from build123d import *

# Parameters (mm, degrees)
SKETCH_1_W          = 20
SKETCH_1_H          = 15
SKETCH_1_W_2        = 18
SKETCH_1_H_2        = 13
EXTRUDE_1_DEPTH     = 200
SKETCH_3_R          = 1.6
CUT_EXTRUDE_1_DEPTH = 202.137390855
SKETCH_4_R          = 1.6
CUT_EXTRUDE_2_DEPTH = 202.137390855


with BuildPart() as part:
    # 草图1 → 拉伸-薄壁1 (new body)
    with BuildSketch(Plane(origin=(0, 0, 0), x_dir=(1, 0, 0), z_dir=(0, 1, 0))):
        Rectangle(SKETCH_1_W, SKETCH_1_H)
        Rectangle(SKETCH_1_W_2, SKETCH_1_H_2, mode=Mode.SUBTRACT)
    extrude(amount=EXTRUDE_1_DEPTH)

    # 草图3 → 切除-拉伸1 (cut, through all)
    with BuildSketch(Plane(origin=(10, 0, 0), x_dir=(0, 0, -1), z_dir=(1, 0, 0))):
        with Locations((-3.75, 142.5)):
            Circle(SKETCH_3_R)
        with Locations((-3.75, 127.5)):
            Circle(SKETCH_3_R)
        with Locations((3.75, 127.5)):
            Circle(SKETCH_3_R)
        with Locations((3.75, 142.5)):
            Circle(SKETCH_3_R)
        with Locations((-3.75, 72.5)):
            Circle(SKETCH_3_R)
        with Locations((3.75, 72.5)):
            Circle(SKETCH_3_R)
        with Locations((3.75, 57.5)):
            Circle(SKETCH_3_R)
        with Locations((-3.75, 57.5)):
            Circle(SKETCH_3_R)
    extrude(amount=-CUT_EXTRUDE_1_DEPTH, mode=Mode.SUBTRACT)

    # 草图4 → 切除-拉伸2 (cut, through all)
    with BuildSketch(Plane(origin=(10, 0, 0), x_dir=(0, 0, -1), z_dir=(1, 0, 0))):
        with Locations((-3.75, 5)):
            Circle(SKETCH_4_R)
        with Locations((-3.75, 15)):
            Circle(SKETCH_4_R)
        with Locations((3.75, 5)):
            Circle(SKETCH_4_R)
        with Locations((3.75, 15)):
            Circle(SKETCH_4_R)
        with Locations((3.75, 185)):
            Circle(SKETCH_4_R)
        with Locations((3.75, 195)):
            Circle(SKETCH_4_R)
        with Locations((-3.75, 185)):
            Circle(SKETCH_4_R)
        with Locations((-3.75, 195)):
            Circle(SKETCH_4_R)
    extrude(amount=-CUT_EXTRUDE_2_DEPTH, mode=Mode.SUBTRACT)


solid = part.part
The model under review builds one solid part; all positions refer to its coordinate system, in mm. A direction names the side the tool comes from. Round coordinates to 2 decimals unless told otherwise and drop trailing zeros. Order: outer loops, then holes, each group sorted by start corner. A loop starts at its lowest first (then second) coordinate and runs counter-clockwise, first axis right, second up. Notation, with made-up numbers: (32, -32.5) -> (77, -32.5) arc R15 cw to (77, -26.5) -> close; hole circle Ø4 at (2.5, 53). An arc over 180 degrees is marked (long way). Write item = value, one per line. Start each with the question number.
Item 1: Consider section A-A on x = -0.5. Write out the cut boundary in (y, z), plus the area to 3 significant figures.
Item 2: For faces 4 (the face through (-9, 99, 0)), 5 (the face through (9.51, 193.58, -4.49)), list the 3-axis set-ups (+Z, -Z, +X, -X, +Y, -Y) from which the entire face can be reached by the end or side of a thin tool; tool diameter is ignored.
Item 3: Clearance check with a flat-ended pin moving along its axis: pin 1 Ø1.9 at (y, z) = (57.5, 3.75) entering from +X. State where the tip first meets the part, or that it passes through.
Item 4: Mouldability with a two-part tool opening along Y and no side actions: class faces 1 (the face through (0, 99, 6.5)), 2 (the face through (9.51, 126.08, -4.49)), 3 (the face through (-1, 200, 7)) as released by +Y, released by -Y, zero draft, split by the parting line, or undercut.
Item 5: For line 1 along Z through (x, y) = (9.55, 72.5); line 2 along X through (y, z) = (123, 5.25); line 3 along Z through (x, y) = (-6.5, 176), list the stretches that pass through material, from the lowest coordinate up.
Item 6: Consider section B-B on y = 27.5. Write out the cut boundary in (x, z), plus the area to 3 significant figures.
Conclusion:
q1.outline = (0, -7.5) -> (200, -7.5) -> (200, -6.5) -> (0, -6.5) -> close; (0, 6.5) -> (200, 6.5) -> (200, 7.5) -> (0, 7.5) -> close
q1.area = 400 mm2
q2.face_4 = +Y, -Y
q2.face_5 = +X, -X
q3.pin_1 = through
q4.face_1 = zero draft
q4.face_2 = undercut
q4.face_3 = released by +Y
q5.line_1 = -7.5 to -5.35, -2.15 to 2.15, 5.35 to 7.5
q5.line_2 = -10 to -9, 9 to 10
q5.line_3 = -7.5 to -6.5, 6.5 to 7.5
q6.outline = (-10, -7.5) -> (10, -7.5) -> (10, 7.5) -> (-10, 7.5) -> close; hole (-9, -6.5) -> (9, -6.5) -> (9, 6.5) -> (-9, 6.5) -> close
q6.area = 66.0 mm2
